Source: CAD feature listing. Evaluate the final solid. Frame: model axes, mm. A direction names the side the tool comes from. Give positions to 0.01 mm unless a question says otherwise; leave off trailing zeros. Loops run counter-clockwise (first coordinate to the right, second up) from the corner with the lowest first, then second, coordinate; pieces in that order, holes last. Notation, with made-up numbers: (58, 9.5) - (88, 9.5) arc R20 cw to (88, 19.5) - close; hole circle Ø6 at (7.25, 12.25). An arc over 180 degrees is marked (long way). Write each question's results on one line, items separated by ' | '. Start each with the question number.
(1) Material intervals for line 1 along X through (y, z) = (11, 2); line 2 along X through (y, z) = (42, 2.45); line 3 along Y through (x, z) = (15, 3), sorted ascending. Write a range as [from, to].
(2) Contact query for flat-ended pins moving along their axis: pin 1 (5.5 mm diameter, centred on y = 60.5, z = -15, fed in from -X); pin 2 (8 mm diameter, centred on y = -7, z = -22, fed in from -X); pin 3 (4 mm diameter, centred on x = -27.5, z = -4.5, fed in from +Y); pin 4 (3.5 mm diameter, centred on x = -37.5, y = 42, fed in from -Z). Output: stop coordinate, or through.
(3) Cut plane C-C on z = -15. Return the cut outline in (x, y).
(4) Pull-direction query (X, two-part tool) for faces 4 (the cylindrical face through (-5.76, 40.58, 2.46)), 5 (the flat face through (27, -4, 3)), 6 (the flat face through (-17, 48, -11)), 7 (the flat face through (-8.5, -30, -11)); classes: pulls with the +X half, pulls with the -X half, needs draft (parallel to the pull), parting line crosses it, or undercut.
(5) Cut plane B-B on y = 42. Return the cut outline in (x, z).
(6) Cut plane A-A on y = 26.5. Return the cut outline in (x, z), then the cut area to 3 significant figures.
(7) Reachability of faces 1 (the flat face through (-22, 0, -8)), 2 (the flat face through (-25.99, 2.46, -13.31)), 3 (the flat face through (-4, -49, -18.1)) from +Z, -Z, +X, -X, +Y, -Y: full face, straight path, thin tool, end or side. Return the list, or none.
(8) Cut plane D-D on x = -12.5. Return the cut outline in (y, z), then the cut area to 3 significant figures.
from build123d import *

# Parameters (mm, degrees)
PAD_DEPTH         = 60
PAD_DEPTH_BACK    = 53
SKETCH001_R       = 11
SKETCH001_R_2     = 1.6
SKETCH001_R_3     = 3.1
SKETCH001_W       = 34.5
SKETCH001_H       = 60
POCKET_DEPTH      = 27.001
POCKET_DEPTH_BACK = -5.001
POCKET001_DEPTH   = 43.001
PAD001_DEPTH      = 5
PAD002_DEPTH      = 5
SKETCH005_W       = 43
SKETCH005_H       = 27
POCKET002_DEPTH   = 43.001
SKETCH006_W       = 8.5
SKETCH006_H       = 32
PAD003_DEPTH      = 15
SKETCH007_R       = 3.1
POCKET003_DEPTH   = 43.001


with BuildPart() as part:
    # Sketch → Pad (new body, two sides)
    with BuildSketch(Plane.XZ) as pad_sk:
        Polygon((-43, 5), (27, 5), (27, 0), (0, 0), (0, -27), (-8.5, -27), (-8.5, 0), (-43, 0), align=None)
    extrude(amount=PAD_DEPTH)
    extrude(pad_sk.sketch, amount=-PAD_DEPTH_BACK)

    # Sketch001 → Pocket (cut, two sides)
    with BuildSketch(Plane.XY) as pocket_sk:
        with Locations((-22, 26.5)):
            Circle(SKETCH001_R)
        with Locations((-37.5, 42)):
            Circle(SKETCH001_R_2)
        with Locations((-6.5, 42)):
            Circle(SKETCH001_R_2)
        with Locations((-37.5, 11)):
            Circle(SKETCH001_R_2)
        with Locations((-6.5, 11)):
            Circle(SKETCH001_R_2)
        with Locations((15, 42)):
            Circle(SKETCH001_R_3)
        with Locations((15, -42)):
            Circle(SKETCH001_R_3)
        with Locations((15, 0)):
            Circle(SKETCH001_R_3)
        with Locations((-25.75, -30)):
            Rectangle(SKETCH001_W, SKETCH001_H)
    extrude(amount=-POCKET_DEPTH, mode=Mode.SUBTRACT)
    extrude(pocket_sk.sketch, amount=-POCKET_DEPTH_BACK, mode=Mode.SUBTRACT)

    # Sketch002 → Pocket001 (cut, through all)
    with BuildSketch(Plane.YZ):
        with BuildLine():
            ThreePointArc((-50, -11.9), (-53.1, -15), (-50, -18.1))
            Line((-50, -18.1), (-47, -18.1))
            ThreePointArc((-47, -18.1), (-43.9, -15), (-47, -11.9))
            Line((-50, -11.9), (-47, -11.9))
        make_face()
        with BuildLine():
            ThreePointArc((-8, -11.9), (-11.1, -15), (-8, -18.1))
            Line((-8, -18.1), (-5, -18.1))
            ThreePointArc((-5, -18.1), (-1.9, -15), (-5, -11.9))
            Line((-8, -11.9), (-5, -11.9))
        make_face()
    extrude(amount=-POCKET001_DEPTH, mode=Mode.SUBTRACT)

    # Sketch003 → Pad001 (join)
    with BuildSketch(Plane.XZ):
        Polygon((-43, 5), (-43, 0), (-8.5, -27), (0, -27), (0, 5), align=None)
    extrude(amount=-PAD001_DEPTH)

    # Sketch004 (on Face1 of Pad001) → Pad002 (join)
    with BuildSketch(Plane(origin=(0, 53, 0), x_dir=(1, 0, 0), z_dir=(0, 1, 0))):
        Polygon((-43, -5), (0, -5), (0, 27), (-8.5, 27), (-43, 0), align=None)
    extrude(amount=-PAD002_DEPTH)

    # Sketch005 → Pocket002 (cut, through all)
    with BuildSketch(Plane.YZ):
        with Locations((26.5, -13.5)):
            Rectangle(SKETCH005_W, SKETCH005_H)
    extrude(amount=-POCKET002_DEPTH, mode=Mode.SUBTRACT)

    # Sketch006 (on Face4 of Pocket002) → Pad003 (join)
    with BuildSketch(Plane(origin=(0, 53, 0), x_dir=(1, 0, 0), z_dir=(0, 1, 0))):
        with Locations((-4.25, 11)):
            Rectangle(SKETCH006_W, SKETCH006_H)
    extrude(amount=PAD003_DEPTH)

    # Sketch007 → Pocket003 (cut, through all)
    with BuildSketch(Plane.YZ):
        with Locations((60.5, -15)):
            Circle(SKETCH007_R)
    extrude(amount=-POCKET003_DEPTH, mode=Mode.SUBTRACT)


solid = part.part
Ans:
1) line 1: [-43, -39.1], [-35.9, -8.1], [-4.9, 27] | line 2: [-43, -39.1], [-35.9, -8.1], [-4.9, 11.9], [18.1, 27] | line 3: [-60, -45.1], [-38.9, -3.1], [3.1, 38.9], [45.1, 53]
2) pin 1: through | pin 2: x = -8.5 | pin 3: y = 53 | pin 4: z = 0
3) outline: (-23.83, 0) - (-8.5, 0) - (-8.5, -1.9) - (0, -1.9) - (0, 5) - (-23.83, 5) - close; (-23.83, 48) - (0, 48) - (0, 57.4) - (-8.5, 57.4) - (-8.5, 53) - (-23.83, 53) - close; (-8.5, -60) - (0, -60) - (0, -53.1) - (-8.5, -53.1) - close; (-8.5, -43.9) - (0, -43.9) - (0, -11.1) - (-8.5, -11.1) - close; (-8.5, 63.6) - (0, 63.6) - (0, 68) - (-8.5, 68) - close
4) face 4: undercut | face 5: pulls with the +X half | face 6: needs draft | face 7: pulls with the -X half
5) outline: (-43, 0) - (-39.1, 0) - (-39.1, 5) - (-43, 5) - close; (-35.9, 0) - (-8.1, 0) - (-8.1, 5) - (-35.9, 5) - close; (-4.9, 0) - (11.9, 0) - (11.9, 5) - (-4.9, 5) - close; (18.1, 0) - (27, 0) - (27, 5) - (18.1, 5) - close
6) outline: (-43, 0) - (-33, 0) - (-33, 5) - (-43, 5) - close; (-11, 0) - (27, 0) - (27, 5) - (-11, 5) - close | area: 240 mm^2
7) face 1: +Z, -Z, -X, -Y | face 2: -Z, -X, +Y, -Y | face 3: +X, -X
8) outline: (0, -23.87) - (5, -23.87) - (5, 0) - (20.95, 0) - (20.95, 5) - (0, 5) - close; (32.05, 0) - (48, 0) - (48, -23.87) - (53, -23.87) - (53, 5) - (32.05, 5) - close | area: 448 mm^2
